The listing builds one solid part. Answer for the finished solid, in the listing's coordinates (mm). Face numbers are marked on the shaded views. A direction names the side the tool comes from. Coordinates: 2 decimals unless noted, no trailing zeros. Write each loop counter-clockwise with the first axis right and the second up, starting at its lowest first coordinate (ties: lowest second). Pieces come first, ordered by that corner, then holes. Notation, with made-up numbers: M 79.25,7 L 120.25,7 A10 ccw 120.25,21 Z; hole C 84.5,-38.5 d10. An arc over 180 degrees is marked long. Answer as CSV lines item,"result". Start each with the question number.
```python
from build123d import *

# Parameters (mm, degrees)
SKETCH1_W            = 2.5
SKETCH1_H            = 1.5
BOSS_EXTRUDE1_DEPTH  = 1.8
SKETCH2_W            = 2.272709172
SKETCH2_H            = 1.309335963
CUT_EXTRUDE1_DEPTH   = 1.7
SKETCH3_W            = 0.001965442
SKETCH3_H            = 0.00266433
SKETCH3_W_2          = 1.44909182
SKETCH3_H_2          = 0.895759853
CUT_EXTRUDE2_DEPTH   = 1.8
SCALE1_SCALE         = 10
SKETCH6_W            = 3.399300392
SKETCH6_H            = 8.946780682
CUT_EXTRUDE4_DEPTH   = 10
SKETCH12_W           = 4.961896536
SKETCH12_H           = 15
BOSS_EXTRUDE5_DEPTH  = 8
SKETCH13_R           = 1.698754484
CUT_EXTRUDE6_DEPTH   = 34
SKETCH22_W           = 12.579678002
SKETCH22_H           = 9.485518979
BOSS_EXTRUDE10_DEPTH = 3
SKETCH25_R           = 1.733474482
CUT_EXTRUDE7_DEPTH   = 36
SKETCH26_W           = 6.246850144
SKETCH26_H           = 18
BOSS_EXTRUDE11_DEPTH = 2
SKETCH27_W           = 6.184798315
SKETCH27_H           = 18
BOSS_EXTRUDE12_DEPTH = 2
SKETCH28_W           = 12.580266047
SKETCH28_H           = 15
BOSS_EXTRUDE13_DEPTH = 2
SKETCH29_W           = 6.217055849
SKETCH29_H           = 18
BOSS_EXTRUDE14_DEPTH = 2
SKETCH30_W           = 6.149592849
SKETCH30_H           = 18
BOSS_EXTRUDE15_DEPTH = 2
SKETCH31_W           = 12.597557791
SKETCH31_H           = 15
BOSS_EXTRUDE16_DEPTH = 2
SKETCH32_W           = 8
SKETCH32_H           = 4.961896536
BOSS_EXTRUDE17_DEPTH = 2
SKETCH33_W           = 0.035793511
SKETCH33_H           = 18
BOSS_EXTRUDE18_DEPTH = 2
SKETCH34_W           = 8
SKETCH34_H           = 4.961896536
BOSS_EXTRUDE19_DEPTH = 2
SKETCH36_W           = 18
SKETCH36_H           = 4.317479632
BOSS_EXTRUDE20_DEPTH = 2
SKETCH37_W           = 18
SKETCH37_H           = 5.630697462
BOSS_EXTRUDE21_DEPTH = 2
SKETCH38_W           = 2.199407661
SKETCH38_H           = 9.051822906
BOSS_EXTRUDE22_DEPTH = 2
SKETCH39_W           = 15.800592339
SKETCH39_H           = 0.042851216
BOSS_EXTRUDE23_DEPTH = 2
SKETCH40_W           = 15.800592339
SKETCH40_H           = 0.062191008
BOSS_EXTRUDE24_DEPTH = 2


with BuildPart() as part:
    # Sketch1 → Boss-Extrude1 (new body)
    with BuildSketch(Plane.XY):
        with Locations((0.15674366, 0.085055811)):
            Rectangle(SKETCH1_W, SKETCH1_H)
    extrude(amount=BOSS_EXTRUDE1_DEPTH)

    # Sketch2 → Cut-Extrude1 (cut)
    with BuildSketch(Plane.XY.offset(1.8)):
        with Locations((0.160861454, 0.075181403)):
            Rectangle(SKETCH2_W, SKETCH2_H)
    extrude(amount=-CUT_EXTRUDE1_DEPTH, mode=Mode.SUBTRACT)

    # Sketch3 → Cut-Extrude2 (cut)
    with BuildSketch(Plane(origin=(1.40674366, 0, 0), x_dir=(0, 0, -1), z_dir=(1, 0, 0))):
        with Locations((-0.29122496, -0.460339146)):
            Rectangle(SKETCH3_W, SKETCH3_H)
        with Locations((-0.943862586, 0.020902802)):
            Rectangle(SKETCH3_W_2, SKETCH3_H_2)
    extrude(amount=-CUT_EXTRUDE2_DEPTH, mode=Mode.SUBTRACT)


with BuildPart() as part_1:
    # Scale1: scaled about (0.033599126, 0.123190455, 0.732690955)
    add(part.part.scale(SCALE1_SCALE).moved(Location((-0.302392134, -1.108714095, -6.594218595))))

    # Sketch6 → Cut-Extrude4 (cut)
    with BuildSketch(Plane(origin=(13.765044467, 0, 0), x_dir=(0, 0, -1), z_dir=(1, 0, 0))):
        with Locations((-11.016576897, -0.905094997)):
            Rectangle(SKETCH6_W, SKETCH6_H)
    extrude(amount=-CUT_EXTRUDE4_DEPTH, mode=Mode.SUBTRACT)

    # Sketch12 → Boss-Extrude5 (add)
    with BuildSketch(Plane.ZY.offset(11.234955533)):
        with Locations((8.924833137, -0.258155978)):
            Rectangle(SKETCH12_W, SKETCH12_H)
    extrude(amount=BOSS_EXTRUDE5_DEPTH)

    # Sketch13 → Cut-Extrude6 (cut)
    with BuildSketch(Plane.XY.offset(11.405781405)):
        with Locations((-13.415722705, 0.071814751)):
            Circle(SKETCH13_R)
    extrude(amount=-CUT_EXTRUDE6_DEPTH, mode=Mode.SUBTRACT)

    # Sketch22 → Boss-Extrude10 (add)
    with BuildSketch(Plane(origin=(0, 0, -6.594218595), x_dir=(-1, 0, 0), z_dir=(0, 0, -1))):
        with Locations((-1.289819106, 11.984603512)):
            Rectangle(SKETCH22_W, SKETCH22_H)
        with Locations((-1.289819106, -12.500915468)):
            Rectangle(SKETCH22_W, SKETCH22_H)
    extrude(amount=-BOSS_EXTRUDE10_DEPTH)

    # Sketch25 → Cut-Extrude7 (cut)
    with BuildSketch(Plane.XY.offset(-3.594218595)):
        with Locations((1.268574204, 12.179653892)):
            Circle(SKETCH25_R)
        with Locations((1.268574204, -12.893454026)):
            Circle(SKETCH25_R)
    extrude(amount=-CUT_EXTRUDE7_DEPTH, mode=Mode.SUBTRACT)

    # Sketch26 → Boss-Extrude11 (add)
    with BuildSketch(Plane(origin=(0, 7.241844022, 0), x_dir=(1, 0, 0), z_dir=(0, 1, 0))):
        with Locations((-8.111530461, -2.405781405)):
            Rectangle(SKETCH26_W, SKETCH26_H)
    extrude(amount=BOSS_EXTRUDE11_DEPTH)

    # Sketch27 → Boss-Extrude12 (add)
    with BuildSketch(Plane(origin=(0, 7.241844022, 0), x_dir=(1, 0, 0), z_dir=(0, 1, 0))):
        with Locations((10.67264531, -2.405781405)):
            Rectangle(SKETCH27_W, SKETCH27_H)
    extrude(amount=BOSS_EXTRUDE12_DEPTH)

    # Sketch28 → Boss-Extrude13 (add)
    with BuildSketch(Plane(origin=(0, 7.241844022, 0), x_dir=(1, 0, 0), z_dir=(0, 1, 0))):
        with Locations((1.290113129, -3.905781405)):
            Rectangle(SKETCH28_W, SKETCH28_H)
    extrude(amount=BOSS_EXTRUDE13_DEPTH)

    # Sketch29 → Boss-Extrude14 (add)
    with BuildSketch(Plane(origin=(0, -7.758155978, 0), x_dir=(-1, 0, 0), z_dir=(0, -1, 0))):
        with Locations((8.126427609, -2.405781405)):
            Rectangle(SKETCH29_W, SKETCH29_H)
    extrude(amount=BOSS_EXTRUDE14_DEPTH)

    # Sketch30 → Boss-Extrude15 (add)
    with BuildSketch(Plane(origin=(0, -7.758155978, 0), x_dir=(-1, 0, 0), z_dir=(0, -1, 0))):
        with Locations((-10.690248043, -2.405781405)):
            Rectangle(SKETCH30_W, SKETCH30_H)
    extrude(amount=BOSS_EXTRUDE15_DEPTH)

    # Sketch31 → Boss-Extrude16 (add)
    with BuildSketch(Plane.XZ.offset(7.758155978)):
        with Locations((1.280879211, 3.905781405)):
            Rectangle(SKETCH31_W, SKETCH31_H)
    extrude(amount=BOSS_EXTRUDE16_DEPTH)

    # Sketch32 → Boss-Extrude17 (add)
    with BuildSketch(Plane(origin=(0, 7.241844022, 0), x_dir=(1, 0, 0), z_dir=(0, 1, 0))):
        with Locations((-15.234955533, -8.924833137)):
            Rectangle(SKETCH32_W, SKETCH32_H)
    extrude(amount=BOSS_EXTRUDE17_DEPTH)

    # Sketch33 → Boss-Extrude18 (add)
    with BuildSketch(Plane(origin=(0, -7.758155978, 0), x_dir=(-1, 0, 0), z_dir=(0, -1, 0))):
        with Locations((-7.597554863, -2.405781405)):
            Rectangle(SKETCH33_W, SKETCH33_H)
    extrude(amount=BOSS_EXTRUDE18_DEPTH)

    # Sketch34 → Boss-Extrude19 (add)
    with BuildSketch(Plane.XZ.offset(7.758155978)):
        with Locations((-15.234955533, 8.924833137)):
            Rectangle(SKETCH34_W, SKETCH34_H)
    extrude(amount=BOSS_EXTRUDE19_DEPTH)

    # Sketch36 → Boss-Extrude20 (add)
    with BuildSketch(Plane(origin=(13.765044467, 0, 0), x_dir=(0, 0, -1), z_dir=(1, 0, 0))):
        with Locations((-2.405781405, -7.599416162)):
            Rectangle(SKETCH36_W, SKETCH36_H)
    extrude(amount=BOSS_EXTRUDE20_DEPTH)

    # Sketch37 → Boss-Extrude21 (add)
    with BuildSketch(Plane(origin=(13.765044467, 0, 0), x_dir=(0, 0, -1), z_dir=(1, 0, 0))):
        with Locations((-2.405781405, 6.426495291)):
            Rectangle(SKETCH37_W, SKETCH37_H)
    extrude(amount=BOSS_EXTRUDE21_DEPTH)

    # Sketch38 → Boss-Extrude22 (add)
    with BuildSketch(Plane(origin=(13.765044467, 0, 0), x_dir=(0, 0, -1), z_dir=(1, 0, 0))):
        with Locations((5.494514764, -0.914764893)):
            Rectangle(SKETCH38_W, SKETCH38_H)
    extrude(amount=BOSS_EXTRUDE22_DEPTH)

    # Sketch39 → Boss-Extrude23 (add)
    with BuildSketch(Plane(origin=(13.765044467, 0, 0), x_dir=(0, 0, -1), z_dir=(1, 0, 0))):
        with Locations((-3.505485236, 3.589720952)):
            Rectangle(SKETCH39_W, SKETCH39_H)
    extrude(amount=BOSS_EXTRUDE23_DEPTH)

    # Sketch40 → Boss-Extrude24 (add)
    with BuildSketch(Plane(origin=(13.765044467, 0, 0), x_dir=(0, 0, -1), z_dir=(1, 0, 0))):
        with Locations((-3.505485236, -5.409580842)):
            Rectangle(SKETCH40_W, SKETCH40_H)
    extrude(amount=BOSS_EXTRUDE24_DEPTH)


solid = part_1.part
```
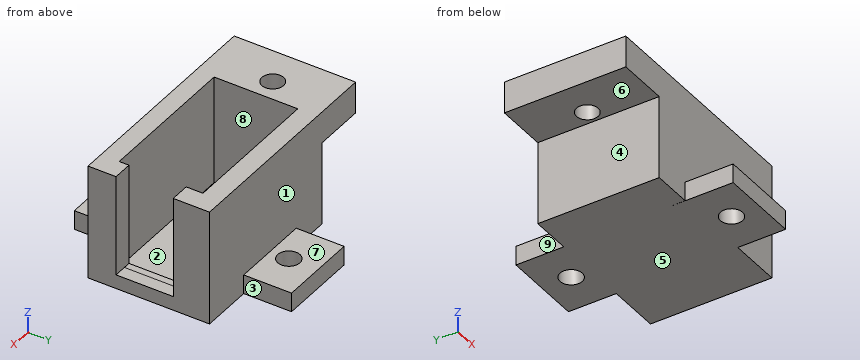
1) For a pull along X with two mould halves and no side action, classify the marked faces 1, 2, 3 and 4 as +X half, -X half, draft (parallel to the pull), parting line (faces both ways), or undercut.
2) The part is cut by section A-A (y = 5). Determine the outline of the cut face in (x, z), then the cut area to 3 significant figures.
3) The part is cut by section B-B (x = 9). Determine the outline of the cut face in (y, z).
4) Each of these flat-tipped pins is pushed along its axis until it touches: P1, Ø3, axis at x = -13, z = 5, coming from the +Y side; P2, Ø1.5, axis at x = -4, y = 2, coming from the +Z side; P3, Ø0.9, axis at y = 13.5, z = -5, coming from the -X side. Where does it stop, or does it pass through?
5) Which of the six approach directions +Z, -Z, +X, -X, +Y, -Y give full straight-line access (tool end or side, diameter ignored) to the marked faces 5, 6, 7, 8 and 9?
6) The part is cut by section D-D (x = -2). Determine the outline of the cut face in (y, z).
7) Find the intervals of material crossed by line 1 (Y direction, x = 10.5, z = 4.5); line 2 (X direction, y = 5, z = 9.75); line 3 (Y direction, x = 7.5, z = -3.75), in increasing order. Write a range as from..to.
Completed:
1,face 1,"draft"
1,face 2,"undercut"
1,face 3,"undercut"
1,face 4,"-X half"
2,outline,"M -19.23,6.44 L -11.23,6.44 L -11.23,-6.59 L 15.77,-6.59 L 15.77,11.41 L 12.67,11.41 L 12.67,-5.59 L -10.06,-5.59 L -10.06,11.41 L -19.23,11.41 Z"
2,area,"139 mm²"
3,outline,"M -9.76,-6.59 L 9.24,-6.59 L 9.24,11.41 L 6.19,11.41 L 6.19,-5.59 L -6.9,-5.59 L -6.9,11.41 L -9.76,11.41 Z"
4,P1,"y = 9.24"
4,P2,"z = -5.59"
4,P3,"x = -5"
5,face 5,"-Z, +X, -X, +Y, -Y"
5,face 6,"-Z, -X, +Y, -Y"
5,face 7,"+Z, +X, -X, +Y"
5,face 8,"+Z"
5,face 9,"+Z, -Z, -X, +Y"
6,outline,"M -17.24,-6.59 L 16.73,-6.59 L 16.73,-3.59 L 9.24,-3.59 L 9.24,11.41 L 6.19,11.41 L 6.19,-5.59 L -6.9,-5.59 L -6.9,11.41 L -9.76,11.41 L -9.76,-3.59 L -17.24,-3.59 Z"
7,line 1,"-9.76..-6.9, 6.19..9.24"
7,line 2,"-19.23..-10.06, 12.67..15.77"
7,line 3,"-17.24..-6.9, 6.19..16.73"
